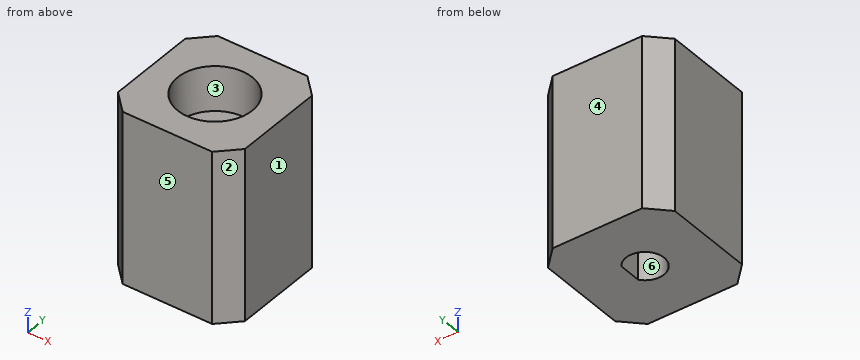
```python
from build123d import *

# Parameters (mm, degrees)
SKETCH3_W           = 17
SKETCH3_H           = 17
BOSS_EXTRUDE1_DEPTH = 23
CUT_EXTRUDE1_DEPTH  = 34.271609519
SKETCH5_R           = 5
CUT_EXTRUDE2_DEPTH  = 6
CUT_EXTRUDE3_DEPTH  = 6


with BuildPart() as part:
    # Sketch3 → Boss-Extrude1 (new body)
    with BuildSketch(Plane.XY):
        with Locations((8.5, -8.5)):
            Rectangle(SKETCH3_W, SKETCH3_H)
    extrude(amount=BOSS_EXTRUDE1_DEPTH)

    # Sketch4 → Cut-Extrude1 (cut, through all)
    with BuildSketch(Plane.XY.offset(23)):
        Polygon((17, 0), (14.5, 0), (17, -2.5), align=None)
        Polygon((0, -2.5), (2.5, 0), (0, 0), align=None)
        Polygon((2.5, -17), (0, -14.5), (0, -17), align=None)
        Polygon((17, -17), (17, -14.5), (14.5, -17), align=None)
    extrude(amount=-CUT_EXTRUDE1_DEPTH, mode=Mode.SUBTRACT)

    # Sketch5 → Cut-Extrude2 (cut)
    with BuildSketch(Plane.XY.offset(23)):
        with Locations((8.5, -8.5)):
            Circle(SKETCH5_R)
    extrude(amount=-CUT_EXTRUDE2_DEPTH, mode=Mode.SUBTRACT)

    # Sketch6 → Cut-Extrude3 (cut)
    with BuildSketch(Plane(origin=(0, 0, 0), x_dir=(-1, 0, 0), z_dir=(0, 0, -1))):
        with BuildLine():
            Line((-10.55, -6.983424911), (-10.55, -10.016575089))
            ThreePointArc((-10.55, -10.016575089), (-5.95, -8.5), (-10.55, -6.983424911))
        make_face()
    extrude(amount=-CUT_EXTRUDE3_DEPTH, mode=Mode.SUBTRACT)


solid = part.part
```
Here's how the part is built. I have some questions about the finished solid (model axes, mm). Face numbers are marked on the shaded views. A direction names the side the tool comes from. Give positions to 0.01 mm unless a question says otherwise; leave off trailing zeros. Loops run counter-clockwise (first coordinate to the right, second up) from the corner with the lowest first, then second, coordinate; pieces in that order, holes last. Notation, with made-up numbers: M 19.25,26.5 L 61.25,26.5 A36 ccw 61.25,65.5 Z; hole C 3,41 d11. An arc over 180 degrees is marked long. Use one line per item in the form item = value. Start each with the question number.
Q1. If we section it at D-D (y = -8.5): Write out the boundary of the cut face in (x, z), then the cut area to 3 significant figures.
Q2. If we section it at B-B (x = 4.5): Write out the boundary of the cut face in (y, z), then the cut area to 3 significant figures.
Q3. Thinking about a two-plate mould opening in Y: for the marked faces 1, 2, 3 and 4, which applies, +Y half, -Y half, draft (parallel to the pull), parting line (faces both ways), or undercut?
Q4. Which directions (+Z, -Z, +X, -X, +Y, -Y) give clear straight access to the entire face, cutting with the end or side of a thin tool? Please do the marked faces 5 and 6.
Q5. Will this pin go through, and if not, where does the flat tip stop? pin 1 Ø4.5 at (x, y) = (8.5, -8.5) entering from +Z.
Q6. I need wall thicknesses on line 1 along Y through (x, z) = (8.5, 4); line 2 along X through (y, z) = (-8.5, 2.7); line 3 along Y through (x, z) = (8.5, 20.85). Which ranges of each line are inside material? Lowest first, please.
Q7. If we section it at A-A (z = 18.5): Write out the boundary of the cut face in (x, y), then the cut area to 3 significant figures.
Q8. If we section it at C-C (z = 14): Write out the boundary of the cut face in (x, y), then the cut area to 4 significant figures.
Taken from the geometry:
q1.outline = M 0,0 L 5.95,0 L 5.95,6 L 10.55,6 L 10.55,0 L 17,0 L 17,23 L 13.5,23 L 13.5,17 L 3.5,17 L 3.5,23 L 0,23 Z
q1.area = 303 mm^2
q2.outline = M -17,0 L 0,0 L 0,23 L -5.5,23 L -5.5,17 L -11.5,17 L -11.5,23 L -17,23 Z
q2.area = 355 mm^2
q3.face_1 = draft
q3.face_2 = -Y half
q3.face_3 = undercut
q3.face_4 = +Y half
q4.face_5 = +Z, -Z, +X, -X, -Y
q4.face_6 = -Z
q5.pin_1 = 17
q6.line_1 = -17 to -11.05, -5.95 to 0
q6.line_2 = 0 to 5.95, 10.55 to 17
q6.line_3 = -17 to -13.5, -3.5 to 0
q7.outline = M 0,-14.5 L 2.5,-17 L 14.5,-17 L 17,-14.5 L 17,-2.5 L 14.5,0 L 2.5,0 L 0,-2.5 Z; hole C 8.5,-8.5 d10
q7.area = 198 mm^2
q8.outline = M 0,-14.5 L 2.5,-17 L 14.5,-17 L 17,-14.5 L 17,-2.5 L 14.5,0 L 2.5,0 L 0,-2.5 Z
q8.area = 276.5 mm^2
